Geometry: final body of the model. Coordinates: model frame, mm. A direction names the side the tool comes from. Coordinates: 2 decimals unless noted, no trailing zeros. Order: outer loops, then holes, each group sorted by start corner. A loop starts at its lowest first (then second) coordinate and runs counter-clockwise, first axis right, second up. Notation, with made-up numbers: (-10, -2) -> (8, -2) arc R35 cw to (8, 32) -> close; hole circle Ø8 at (72, 88.5). An arc over 180 degrees is marked (long way). Answer in a Markdown table with one row per item. Add a question column.
1) Section query C-C on x = 91.5. Return the cut outline in (y, z) (3 decimals).
2) Ray query, line 1 (X direction, y = -2.5, z = -68.5); line 2 (Y direction, x = 93, z = -67.5); line 3 (Z direction, x = 95.5, y = 1.25). Return the intervals inside material, ascending. Write a range as from..to.
3) Contact query for flat-ended pins moving along their axis: P1, Ø1, axis at x = 90.5, y = -3, coming from the -Z side; P2, Ø2.5, axis at y = -1, z = -68, coming from the -X side; P3, Ø2.5, axis at y = 0, z = -67.5, coming from the -X side. Output: stop coordinate, or through.
4) Section query A-A on y = 0. Return the cut outline in (x, z), then the cut area to 3 significant figures.
5) Set-up query: faces 4 (the face through (92.501, 3, -68)), 5 (the face through (95.501, -0.601, -68.325)), 6 (the face through (96.01, -0.13, -63.42)). Return all of +Z, -Z, +X, -X, +Y, -Y with unobstructed straight access to the full face (end or side cutting, diameter ignored); none if empty.
6) Section query B-B on x = 97.25. Return the cut outline in (y, z).
7) Pull-direction query (Y, two-part tool) for faces 1 (the face through (89.994, -1.201, -70.233)), 2 (the face through (90.501, 3, -68)), 3 (the face through (90.733, 0.788, -63.914)); classes: +Y half, -Y half, draft (parallel to the pull), parting line (faces both ways), or undercut.
Autodesk Inventor part; units mm, degrees
ref_plane "YZ Plane" through (0, 0, 0) normal (1, 0, 0) x (0, 1, 0)
ref_plane "XZ Plane" through (0, 0, 0) normal (0, 1, 0) x (-1, 0, 0)
ref_plane "XY Plane" through (0, 0, 0) normal (0, 0, 1) x (1, 0, 0)
sketch "Boceto2" plane through (0, 0, 0) normal (0, 1, 0) x (-1, 0, 0)
  line L0 (99.3538, -66.4173) -> (-152.1277, -66.4173)
  line L1 (-90.5006, -68.4173) -> (-90.5006, -69.4173)
  line L2 (-89.5006, -69.4173) -> (-89.5006, -68.4173)
  line L3 (-92.5006, -68.4173) -> (-92.5006, -69.4173)
  line L4 (-99.1006, -68.4173) -> (-99.1006, -69.4173)
  line L5 (-99.1006, -69.4173) -> (-93.5006, -69.4173)
  line L6 (-93.5006, -70.4173) -> (-92.5006, -70.4173)
  line L7 (-92.5006, -70.4173) -> (-92.5006, -69.4173)
  line L8 (-90.5006, -69.4173) -> (-90.5006, -70.4173)
  line L9 (-90.5006, -70.4173) -> (-89.5006, -70.4173)
  line L10 (-89.5006, -70.4173) -> (-89.5006, -69.4173)
  line L11 (-93.5006, -68.4173) -> (-93.5006, -70.4173)
  line L12 (-92.5006, -69.4173) -> (-90.5006, -69.4173)
  line L13 (-99.1006, -68.4173) -> (-89.5006, -68.4173)
  point P0 (0, 0)
  dimension "d17" = 1
revolve "Revolución1" add sketch "Boceto2" angle 360 about axis through (-99.3538, 0, -66.4173) along (1, 0, 0)
chamfer "Chaflán2" distance 0.5 angle 45 1 edges at (99.1006, 0, -63.4173)
sketch "Boceto3" plane through (89.5006, 0, -66.4173) normal (-1, 0, 0) x (0, 0, 1)
  circle A0 centre (0, 0) radius 2.625
  point P0 (66.4173, 0)
  dimension "d28" = 5.25
extrude "Extrusión3" cut sketch "Boceto3" against normal blind 2.5
thread "Rosca3"
properties part number "Tuerca remache m4" material "Aluminum 7175 T73 0 Hot Formed"
Result:
| question | item | result |
|---|---|---|
| 1 | outline | circle Ø6 at (0, -66.417); hole circle Ø5.25 at (0, -66.417) |
| 2 | line 1 | 89.5..90.5, 92.5..93.5 |
| 2 | line 2 | -3.85..-1.68, 1.68..3.85 |
| 2 | line 3 | -69.14..-67.98, -64.86..-63.69 |
| 3 | P1 | z = -69.54 |
| 3 | P2 | x = 89.5 |
| 3 | P3 | x = 92 |
| 4 | outline | (89.5, -70.42) -> (90.5, -70.42) -> (90.5, -69.42) -> (92.5, -69.42) -> (92.5, -70.42) -> (93.5, -70.42) -> (93.5, -69.42) -> (98.6, -69.42) -> (99.1, -68.92) -> (99.1, -68.42) -> (92, -68.42) -> (92, -69.04) -> (89.5, -69.04) -> close; (89.5, -63.79) -> (92, -63.79) -> (92, -64.42) -> (99.1, -64.42) -> (99.1, -63.92) -> (98.6, -63.42) -> (93.5, -63.42) -> (93.5, -62.42) -> (92.5, -62.42) -> (92.5, -63.42) -> (90.5, -63.42) -> (90.5, -62.42) -> (89.5, -62.42) -> close |
| 4 | area | 19.8 mm2 |
| 5 | face 4 | none |
| 5 | face 5 | +X, -X |
| 5 | face 6 | +X |
| 6 | outline | circle Ø6 at (0, -66.42); hole circle Ø4 at (0, -66.42) |
| 7 | face 1 | parting line |
| 7 | face 2 | draft |
| 7 | face 3 | undercut |
